Work out the finished part from the listing and answer in its coordinate system (mm). A direction names the side the tool comes from. Round coordinates to 2 decimals unless told otherwise and drop trailing zeros. Order: outer loops, then holes, each group sorted by start corner. A loop starts at its lowest first (then second) coordinate and runs counter-clockwise, first axis right, second up. Notation, with made-up numbers: (25, 72.25) - (50, 72.25) arc R17 cw to (50, 89.25) - close; hole circle Ø3 at (-15, 73.25). An arc over 180 degrees is marked (long way). Answer in a Markdown table with one row per item.
from build123d import *

# Parameters (mm, degrees)
F1_DEPTH = 63.5
F0_W     = 26.635827
F0_H     = 19.05
F2_DEPTH = 25.4
F3_DEPTH = 7.9375
F5_DEPTH = 4.7625


with BuildPart() as f1:
    # F0 (on Front) → F1 (new body, symmetric)
    with BuildSketch(Plane.XZ):
        Polygon((-41.275, 9.525), (-41.275, -9.525), (41.275, -9.525), (41.275, 9.525), (22.225, 9.525), align=None)
    extrude(amount=F1_DEPTH, both=True)

    # F0 (on Front) → F2 (join, symmetric)
    with BuildSketch(Plane.XZ):
        with BuildLine():
            Line((22.225, 9.525), (41.275, 9.525))
            Line((41.275, 9.525), (41.275, 27.0002))
            ThreePointArc((41.275, 27.0002), (45.92468, 38.22552), (57.15, 42.8752))
            Line((57.15, 42.8752), (60.325, 42.8752))
            Line((60.325, 42.8752), (60.325, 61.9252))
            Line((60.325, 61.9252), (57.15, 61.9252))
            add(Edge.make_bspline(
                [(54.920282, 61.853951), (55.666465, 61.878241), (56.409811, 61.90192), (57.15, 61.9252)],
                knots=[109.619199, 109.619199, 109.619199, 109.619199, 111.504536, 111.504536, 111.504536, 111.504536], degree=3))
            ThreePointArc((54.920282, 61.853951), (31.678167, 50.894579), (22.225, 27.0002))
            Line((22.225, 27.0002), (22.225, 9.525))
        make_face()
        with Locations((73.642913, 52.4002)):
            Rectangle(F0_W, F0_H)
    extrude(amount=F2_DEPTH, both=True)

    # F0 (on Front) → F3 (join, symmetric)
    with BuildSketch(Plane.XZ):
        with BuildLine():
            add(Edge.make_bspline(
                [(-41.275, 9.525), (-41.442102, 56.961897), (11.534948, 60.441653), (54.920282, 61.853951)],
                knots=[0, 0, 0, 0, 109.619199, 109.619199, 109.619199, 109.619199], degree=3))
            Line((-41.275, 9.525), (22.225, 9.525))
            Line((22.225, 9.525), (22.225, 27.0002))
            ThreePointArc((22.225, 27.0002), (31.678167, 50.894579), (54.920282, 61.853951))
        make_face()
    extrude(amount=F3_DEPTH, both=True)

    # F4 (on face) → F5 (join)
    with BuildSketch(Plane.XY.offset(61.9252)):
        with BuildLine():
            Line((86.960827, -25.4), (86.960827, 25.4))
            ThreePointArc((86.960827, 25.4), (61.560827, 0), (86.960827, -25.4))
        make_face()
        with BuildLine():
            ThreePointArc((86.960827, -25.4), (104.921339, -17.960512), (112.360827, 0))
            ThreePointArc((112.360827, 0), (104.921339, 17.960512), (86.960827, 25.4))
            Line((86.960827, 25.4), (86.960827, -25.4))
        make_face()
    extrude(amount=F5_DEPTH)


solid = f1.part
1) Each of these flat-tipped pins is pushed along its axis until it touches: pin 1 (15.5 mm diameter, centred on x = 8.5, z = 29.5, fed in from -Y); pin 2 (8.5 mm diameter, centred on y = 12.5, z = 16.5, fed in from -X) (3 decimals); pin 3 (2 mm diameter, centred on x = 79, z = 54.5, fed in from +Y); pin 4 (2 mm diameter, centred on x = 44, y = 49, fed in from -Z). Where does it stop, or does it pass through?
Filled in:
| item | result |
|---|---|
| pin 1 | stops at y = -7.94 |
| pin 2 | stops at x = 22.225 |
| pin 3 | stops at y = 25.4 |
| pin 4 | passes through |
2) Find section B-B, the plane z = -0.5. Give the vertices of the cut face in (x, y) (3 decimals).
Filled in:
| item | result |
|---|---|
| outline | (-41.275, -63.5) - (41.275, -63.5) - (41.275, 63.5) - (-41.275, 63.5) - close |
3) Which of the six approach directions +Z, -Z, +X, -X, +Y, -Y give full straight-line access (tool end or side, diameter ignored) to faces 1 (the face through (41.275, -1, 4)), 2 (the face through (47, 25.4, 42)), 3 (the face through (-3, 7.938, 36)), 4 (the face through (47, -25.4, 42))?
Filled in:
| item | result |
|---|---|
| face 1 | -Z, +X, +Y, -Y |
| face 2 | +Z, +X, -X, +Y |
| face 3 | +Z, -X, +Y |
| face 4 | +Z, +X, -X, -Y |
4) Find the intervals of material crossed by probe 1 along Z at (x, y) = (-33.5, 16) (3 decimals); probe 2 along Z at (x, y) = (61, 22); probe 3 along Y at (x, z) = (37.5, 34.5), in increasing order. Write a range as from..to.
Filled in:
| item | result |
|---|---|
| probe 1 | z = -9.525..9.525 |
| probe 2 | z = 42.88..61.93 |
| probe 3 | y = -25.4..25.4 |
5) Find section D-D, the plane x = 83.5. Give the vertices of the cut face in (y, z), then the cut area to 3 significant figures.
Filled in:
| item | result |
|---|---|
| outline | (-25.4, 42.88) - (25.4, 42.88) - (25.4, 61.93) - (25.16, 61.93) - (25.16, 66.69) - (-25.16, 66.69) - (-25.16, 61.93) - (-25.4, 61.93) - close |
| area | 1,210 mm^2 |
6) Find section C-C, the plane y = -41. Give the vertices of the cut face in (x, z) (3 decimals).
Filled in:
| item | result |
|---|---|
| outline | (-41.275, -9.525) - (41.275, -9.525) - (41.275, 9.525) - (-41.275, 9.525) - close |
7) Find section A-A, the plane x = 64. Give the vertices of the cut face in (y, z), then the cut area to 3 significant figures.
Filled in:
| item | result |
|---|---|
| outline | (-25.4, 42.88) - (25.4, 42.88) - (25.4, 61.93) - (10.86, 61.93) - (10.86, 66.69) - (-10.86, 66.69) - (-10.86, 61.93) - (-25.4, 61.93) - close |
| area | 1,070 mm^2 |
